Read the model definition and answer for the solid it produces. Units are mm, in the model's axes. Face numbers are marked on the shaded views. Round coordinates to 2 decimals unless told otherwise and drop trailing zeros. Loops run counter-clockwise (first coordinate to the right, second up) from the corner with the lowest first, then second, coordinate; pieces in that order, holes last. Notation, with made-up numbers: M 20.25,-30.75 L 54.25,-30.75 A26 cw 54.25,-10.75 Z; hole C 2,-6.75 d9. An arc over 180 degrees is marked long. Write each question's results on one line, items separated by ' | '.
```python
from build123d import *

# Parameters (mm, degrees)
SKETCH1_W           = 440
SKETCH1_H           = 175
SKETCH1_R           = 3.25
SKETCH1_R_2         = 9.6
SKETCH1_R_3         = 2.6
SKETCH1_R_4         = 11
BOSS_EXTRUDE1_DEPTH = 3


with BuildPart() as part:
    # Sketch1 → Boss-Extrude1 (new body)
    with BuildSketch(Plane(origin=(0, 0, 0), x_dir=(1, 0, 0), z_dir=(0, 1, 0))):
        with Locations((220, 87.5)):
            Rectangle(SKETCH1_W, SKETCH1_H)
        with Locations(Location((10, 10, 0), (0, 0, 270))):
            Circle(SKETCH1_R, mode=Mode.SUBTRACT)
        with Locations(Location((10, 165, 0), (0, 0, 270))):
            Circle(SKETCH1_R, mode=Mode.SUBTRACT)
        with Locations(Location((430, 165, 0), (0, 0, 270))):
            Circle(SKETCH1_R, mode=Mode.SUBTRACT)
        with Locations(Location((430, 10, 0), (0, 0, 270))):
            Circle(SKETCH1_R, mode=Mode.SUBTRACT)
        with Locations(Location((33, 31.25, 0), (0, 0, 270))):
            Circle(SKETCH1_R_2, mode=Mode.SUBTRACT)
        with Locations(Location((33, 53.75, 0), (0, 0, 270))):
            Circle(SKETCH1_R_2, mode=Mode.SUBTRACT)
        with Locations(Location((33, 76.25, 0), (0, 0, 270))):
            Circle(SKETCH1_R_2, mode=Mode.SUBTRACT)
        with Locations(Location((33, 98.75, 0), (0, 0, 270))):
            Circle(SKETCH1_R_2, mode=Mode.SUBTRACT)
        with Locations(Location((33, 121.25, 0), (0, 0, 270))):
            Circle(SKETCH1_R_2, mode=Mode.SUBTRACT)
        with Locations(Location((33, 143.75, 0), (0, 0, 270))):
            Circle(SKETCH1_R_2, mode=Mode.SUBTRACT)
        with Locations(Location((58, 31.25, 0), (0, 0, 270))):
            Circle(SKETCH1_R_3, mode=Mode.SUBTRACT)
        with Locations(Location((58, 53.75, 0), (0, 0, 270))):
            Circle(SKETCH1_R_3, mode=Mode.SUBTRACT)
        with Locations(Location((58, 76.25, 0), (0, 0, 270))):
            Circle(SKETCH1_R_3, mode=Mode.SUBTRACT)
        with Locations(Location((58, 98.75, 0), (0, 0, 270))):
            Circle(SKETCH1_R_3, mode=Mode.SUBTRACT)
        with Locations(Location((58, 121.25, 0), (0, 0, 270))):
            Circle(SKETCH1_R_3, mode=Mode.SUBTRACT)
        with Locations(Location((58, 143.75, 0), (0, 0, 270))):
            Circle(SKETCH1_R_3, mode=Mode.SUBTRACT)
        with Locations(Location((69.25, 31.25, 0), (0, 0, 270))):
            Circle(SKETCH1_R_3, mode=Mode.SUBTRACT)
        with Locations(Location((69.25, 53.75, 0), (0, 0, 270))):
            Circle(SKETCH1_R_3, mode=Mode.SUBTRACT)
        with Locations(Location((69.25, 76.25, 0), (0, 0, 270))):
            Circle(SKETCH1_R_3, mode=Mode.SUBTRACT)
        with Locations(Location((69.25, 98.75, 0), (0, 0, 270))):
            Circle(SKETCH1_R_3, mode=Mode.SUBTRACT)
        with Locations(Location((69.25, 121.25, 0), (0, 0, 270))):
            Circle(SKETCH1_R_3, mode=Mode.SUBTRACT)
        with Locations(Location((69.25, 143.75, 0), (0, 0, 270))):
            Circle(SKETCH1_R_3, mode=Mode.SUBTRACT)
        with Locations(Location((80.5, 31.25, 0), (0, 0, 270))):
            Circle(SKETCH1_R_3, mode=Mode.SUBTRACT)
        with Locations(Location((80.5, 53.75, 0), (0, 0, 270))):
            Circle(SKETCH1_R_3, mode=Mode.SUBTRACT)
        with Locations(Location((80.5, 76.25, 0), (0, 0, 270))):
            Circle(SKETCH1_R_3, mode=Mode.SUBTRACT)
        with Locations(Location((80.5, 98.75, 0), (0, 0, 270))):
            Circle(SKETCH1_R_3, mode=Mode.SUBTRACT)
        with Locations(Location((80.5, 121.25, 0), (0, 0, 270))):
            Circle(SKETCH1_R_3, mode=Mode.SUBTRACT)
        with Locations(Location((80.5, 143.75, 0), (0, 0, 270))):
            Circle(SKETCH1_R_3, mode=Mode.SUBTRACT)
        with Locations(Location((400, 135, 0), (0, 0, 270))):
            Circle(SKETCH1_R_4, mode=Mode.SUBTRACT)
        with Locations(Location((340, 135, 0), (0, 0, 270))):
            Circle(SKETCH1_R_4, mode=Mode.SUBTRACT)
        with Locations(Location((300, 135, 0), (0, 0, 270))):
            Circle(SKETCH1_R_4, mode=Mode.SUBTRACT)
        with Locations(Location((260, 135, 0), (0, 0, 270))):
            Circle(SKETCH1_R_4, mode=Mode.SUBTRACT)
        with Locations(Location((140, 135, 0), (0, 0, 270))):
            Circle(SKETCH1_R_4, mode=Mode.SUBTRACT)
        with Locations(Location((408, 31.25, 0), (0, 0, 270))):
            Circle(SKETCH1_R_3, mode=Mode.SUBTRACT)
        with Locations(Location((396, 31.25, 0), (0, 0, 270))):
            Circle(SKETCH1_R_3, mode=Mode.SUBTRACT)
        with Locations(Location((384, 31.25, 0), (0, 0, 270))):
            Circle(SKETCH1_R_3, mode=Mode.SUBTRACT)
        with Locations(Location((408, 53.75, 0), (0, 0, 270))):
            Circle(SKETCH1_R_3, mode=Mode.SUBTRACT)
        with Locations(Location((396, 53.75, 0), (0, 0, 270))):
            Circle(SKETCH1_R_3, mode=Mode.SUBTRACT)
        with Locations(Location((384, 53.75, 0), (0, 0, 270))):
            Circle(SKETCH1_R_3, mode=Mode.SUBTRACT)
        with Locations(Location((408, 76.25, 0), (0, 0, 270))):
            Circle(SKETCH1_R_3, mode=Mode.SUBTRACT)
        with Locations(Location((396, 76.25, 0), (0, 0, 270))):
            Circle(SKETCH1_R_3, mode=Mode.SUBTRACT)
        with Locations(Location((384, 76.25, 0), (0, 0, 270))):
            Circle(SKETCH1_R_3, mode=Mode.SUBTRACT)
    extrude(amount=BOSS_EXTRUDE1_DEPTH)


solid = part.part
```
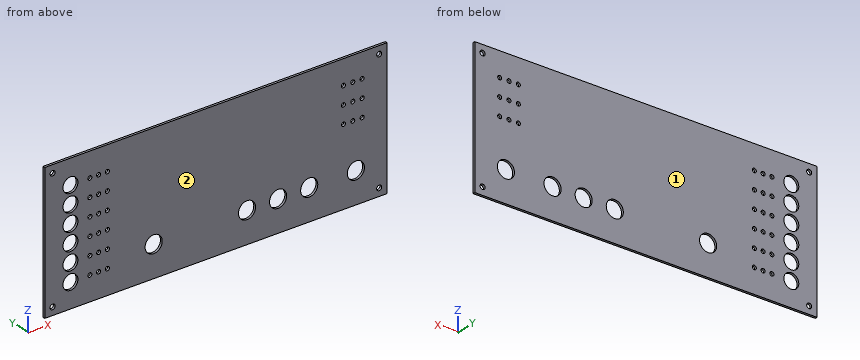
1. Find section B-B, the plane y = 1.7. Count the separate pieces of the cut face and the enclosed holes in it, then the cut area to 3 significant figures.
Completed:
separate pieces: 1 | enclosed holes: 42 | area: 72,700 mm2
2. Determine the mould class of the marked faces 1 and 2 for opening direction Y: released by +Y, released by -Y, zero draft, split by the parting line, or undercut.
Completed:
face 1: released by +Y | face 2: released by -Y
3. Find the intervals of material crossed by L1, parallel to X at y = 1.45, z = -121.25; L2, parallel to Z at x = 384, y = 1.3; L3, parallel to X at y = 0.6, z = -9.5, in increasing order.
Completed:
L1: x = 0 to 23.4, 42.6 to 55.4, 60.6 to 66.65, 71.85 to 77.9, 83.1 to 440 | L2: z = -175 to -78.85, -73.65 to -56.35, -51.15 to -33.85, -28.65 to 0 | L3: x = 0 to 6.79, 13.21 to 426.79, 433.21 to 440
4. Find section A-A, the plane x = 145. Give the vertices of the cut face in (y, z), then the cut area to 3 significant figures.
Completed:
outline: M 0,-175 L 3,-175 L 3,-144.8 L 0,-144.8 Z; M 0,-125.2 L 3,-125.2 L 3,0 L 0,0 Z | area: 466 mm2
